The listing builds one solid part. Answer for the finished solid, in the listing's coordinates (mm). A direction names the side the tool comes from. Give positions to 0.01 mm unless a question says otherwise; leave off trailing zeros. Order: outer loops, then holes, each group sorted by start corner. A loop starts at its lowest first (then second) coordinate and runs counter-clockwise, first axis right, second up. Notation, with made-up numbers: (5, 8.5) - (9, 8.5) arc R30 cw to (9, 32.5) - close; hole circle Ø4 at (1.5, 50). An arc over 180 degrees is marked (long way). Answer in a Markdown table with one row per item.
Autodesk Inventor part; units mm, degrees
ref_plane "YZ Plane" through (0, 0, 0) normal (1, 0, 0) x (0, 1, 0)
ref_plane "XZ Plane" through (0, 0, 0) normal (0, 1, 0) x (-1, 0, 0)
ref_plane "XY Plane" through (0, 0, 0) normal (0, 0, 1) x (1, 0, 0)
sketch "Sketch1" plane through (0, 0, 0) normal (0, 1, 0) x (-1, 0, 0)
  circle A0 centre (0, 0) radius 5
  dimension "d0" = 10
extrude "Extrusion1" add sketch "Sketch1" along normal blind 23
sketch "Sketch2" plane through (0, 23, 0) normal (0, 1, 0) x (1, 0, 0)
  circle A0 centre (0, 0) radius 3
  dimension "d3" = 6
extrude "Extrusion2" add sketch "Sketch2" along normal blind 20
thread "Thread1"
fillet "Fillet1" radius 0.5 1 edges at (-3, 43, 0)
sketch "Sketch3" plane through (0, 0, 0) normal (0, -1, 0) x (1, 0, 0)
  line L0 (4.5, 0) -> (-4.5, 0) construction
  circle A0 centre (0, 0) radius 5
  line L1 (4.5, -2.1794) -> (4.5, 2.1794)
  line L2 (-4.5, -2.1794) -> (-4.5, 2.1794)
extrude "Extrusion3" cut sketch "Sketch3" against normal blind 10 contours A0 L1 | L2 A0
sketch "Sketch4" plane through (0, 0, 0) normal (0, -1, 0) x (1, 0, 0)
  line L0 (3.705, 0) -> (-3.8794, 0) construction
  point P0 (0, 0)
hole "Hole1" at (0, 0, 0) direction (0, 1, 0) diameter 5 depth 14 tip angle 118
properties part number "Semi albero F"
Item 1: Which of the six approach directions +Z, -Z, +X, -X, +Y, -Y give full straight-line access (tool end or side, diameter ignored) to faces 4 (the face through (-4.5, 5, 0)), 5 (the face through (4.5, 5, 0)), 6 (the face through (2, 0, 2))?
Answer block:
| item | result |
|---|---|
| face 4 | +Z, -Z, -X, -Y |
| face 5 | +Z, -Z, +X, -Y |
| face 6 | +Z, -Z, +X, -X, -Y |
Item 2: Find section B-B on y = 24.5. Write down the section's boundary in (x, z), then the cut area to 3 significant figures.
Answer block:
| item | result |
|---|---|
| outline | circle Ø6 at (0, 0) |
| area | 28.3 mm² |
Item 3: Each of these flat-tipped pins is pushed along its axis until it touches: P1, Ø5, axis at y = 14.5, z = -3.5, coming from the -X side; P2, Ø1.3, axis at y = 5.5, z = 0, coming from the -X side; P3, Ø1.3, axis at y = 3.5, z = 0.5, coming from the +X side. Where does it stop, or does it pass through?
Answer block:
| item | result |
|---|---|
| P1 | x = -4.9 |
| P2 | x = -4.5 |
| P3 | x = 4.5 |
Item 4: Consider line 1 (Z direction, x = 0, y = 8.25); line 2 (X direction, y = 4.5, z = 0). Determine where each line is inside the solid, lowest interval first.
Answer block:
| item | result |
|---|---|
| line 1 | -5 to -2.5, 2.5 to 5 |
| line 2 | -4.5 to -2.5, 2.5 to 4.5 |
Item 5: Determine the mould class of faces 1 (the face through (-3, 33, 0)), 2 (the face through (2.44, 7.1, 0.54)), 3 (the face through (-3.3, 23, 0.1)) for opening direction Z: pulls with the +Z half, pulls with the -Z half, needs draft (parallel to the pull), parting line crosses it, or undercut.
Answer block:
| item | result |
|---|---|
| face 1 | parting line crosses it |
| face 2 | undercut |
| face 3 | needs draft |
Item 6: Find section C-C on x = 3.75. Write down the section's boundary in (y, z).
Answer block:
| item | result |
|---|---|
| outline | (0, -3.31) - (23, -3.31) - (23, 3.31) - (0, 3.31) - close |
Item 7: Find section D-D on z = 4.25. Write down the section's boundary in (x, y).
Answer block:
| item | result |
|---|---|
| outline | (-2.63, 0) - (2.63, 0) - (2.63, 23) - (-2.63, 23) - close |
Item 8: Find section A-A on y = 13.5. Write down the section's boundary in (x, z).
Answer block:
| item | result |
|---|---|
| outline | circle Ø10 at (0, 0); hole circle Ø5 at (0, 0) |
